Check sheet for the modelled part. Datum: model origin and axes. Units: mm. A direction names the side the tool comes from. Give positions to 0.01 mm unless a question says otherwise; leave off trailing zeros. Order: outer loops, then holes, each group sorted by start corner. A loop starts at its lowest first (then second) coordinate and runs counter-clockwise, first axis right, second up.
from build123d import *

# Parameters (mm, degrees)
F0_R          = 12.5
F1_DEPTH      = 16
F2_R          = 12.5
F3_DEPTH      = 8
F3_DEPTH_BACK = 8
F5_DEPTH      = 16


with BuildPart() as f1:
    # F0 (on Top) → F1 (new body)
    with BuildSketch(Plane.XY):
        Circle(F0_R)
    extrude(amount=F1_DEPTH)

    # F2 (on Front) → F3 (join, two sides)
    with BuildSketch(Plane.XZ) as f3_sk:
        with Locations((0, 16)):
            Circle(F2_R)
    extrude(amount=F3_DEPTH)
    extrude(f3_sk.sketch, amount=-F3_DEPTH_BACK)

    # F4 (on Top) → F5 (join)
    with BuildSketch(Plane.XY):
        with BuildLine():
            Line((-12.5, 8), (12.5, 8))
            ThreePointArc((12.5, 8), (0, 20.5), (-12.5, 8))
        make_face()
        with BuildLine():
            Line((12.5, -8), (12.5, 8))
            ThreePointArc((12.5, 8), (11.7539052968, 3.7460947032), (9.6046863561, 0))
            ThreePointArc((9.6046863561, 0), (11.7539052968, -3.7460947032), (12.5, -8))
        make_face()
        with BuildLine():
            ThreePointArc((9.6046863561, 0), (11.7539052968, 3.7460947032), (12.5, 8))
            Line((12.5, 8), (-12.5, 8))
            ThreePointArc((-12.5, 8), (-11.7539052968, 3.7460947032), (-9.6046863561, 0))
            ThreePointArc((-9.6046863561, 0), (0, 4.5), (9.6046863561, 0))
        make_face()
        with BuildLine():
            ThreePointArc((-9.6046863561, 0), (-11.7539052968, 3.7460947032), (-12.5, 8))
            Line((-12.5, 8), (-12.5, -8))
            ThreePointArc((-12.5, -8), (-11.7539052968, -3.7460947032), (-9.6046863561, 0))
        make_face()
        with BuildLine():
            ThreePointArc((12.5, -8), (11.7539052968, -3.7460947032), (9.6046863561, 0))
            ThreePointArc((9.6046863561, 0), (0, -4.5), (-9.6046863561, 0))
            ThreePointArc((-9.6046863561, 0), (-11.7539052968, -3.7460947032), (-12.5, -8))
            Line((-12.5, -8), (12.5, -8))
        make_face()
        with BuildLine():
            ThreePointArc((-12.5, -8), (0, -20.5), (12.5, -8))
            Line((12.5, -8), (-12.5, -8))
        make_face()
    extrude(amount=F5_DEPTH)


solid = f1.part
1) Section check D-D, the plane x = 7.25. Record the cut outline in (y, z).
Recorded:
outline: (-18.18, 0) - (18.18, 0) - (18.18, 16) - (8, 16) - (8, 26.18) - (-8, 26.18) - (-8, 16) - (-18.18, 16) - close
2) Material ranges on L1, parallel to Z at x = -9.5, y = 12.5; L2, parallel to Y at x = 0, z = 14.75; L3, parallel to Y at x = -8.25, z = 19, recorded low to high.
Recorded:
L1: z = 0 to 16
L2: y = -20.5 to 20.5
L3: y = -8 to 8
3) Set-up check for faces 1 (the face through (0, 13, 16)), 2 (the face through (0, -8, 21)), 3 (the face through (0, 0, 0)): record each of +Z, -Z, +X, -X, +Y, -Y from which the full face is reachable in a straight line by a thin tool's end or side.
Recorded:
face 1: +Z, +X, -X, +Y
face 2: +Z, +X, -X, -Y
face 3: -Z, +X, -X, +Y, -Y
4) Section check C-C, the plane y = -6. Record the cut outline in (x, z), then the cut area to 3 significant figures.
Recorded:
outline: (-12.5, 0) - (12.5, 0) - (12.5, 16) arc R12.5 ccw to (-12.5, 16) - close
area: 645 mm2
5) Section check A-A, the plane x = 0. Record the cut outline in (y, z).
Recorded:
outline: (-20.5, 0) - (20.5, 0) - (20.5, 16) - (8, 16) - (8, 28.5) - (-8, 28.5) - (-8, 16) - (-20.5, 16) - close
6) Section check B-B, the plane z = 14.5. Record the cut outline in (x, y), then the cut area to 3 significant figures.
Recorded:
outline: (-12.5, -8) arc R12.5 ccw to (12.5, -8) - (12.5, 8) arc R12.5 ccw to (-12.5, 8) - close
area: 891 mm2
7) Depth check by flat-ended pin: pin 1 Ø8 at (y, z) = (-15, 6) entering from +X; pin 2 Ø6 at (x, z) = (3, 25) entering from -Y; pin 3 Ø2 at (x, z) = (-6.5, 7) entering from -Y (3 decimals); pin 4 Ø10 at (y, z) = (-15.5, 24.5) entering from -X. Enter the tip coordinate at first touch or a pass-through.
Recorded:
pin 1: stops at x = 12.13
pin 2: stops at y = -8
pin 3: stops at y = -19.225
pin 4: passes through
